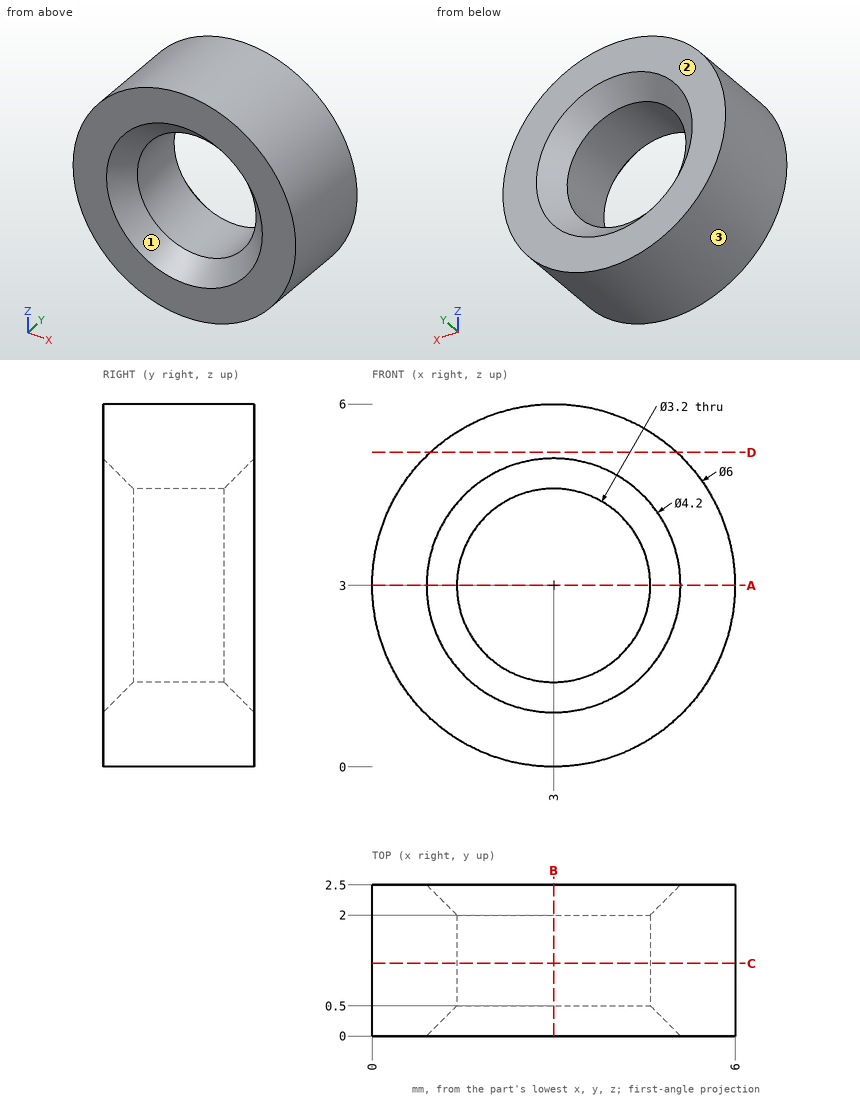
Source: three-view drawing plus pictorial views. Frame: mm from the lowest corner of the part. Give positions to 0.01 mm unless a question says otherwise; leave off trailing zeros. Write each loop counter-clockwise with the first axis right and the second up, starting at its lowest first coordinate (ties: lowest second). Pieces come first, ordered by that corner, then holes.
(1) Ray query, line 1 (Z direction, x = 3, y = 1.3); line 2 (X direction, y = 2.1, z = 2.15); line 3 (Z direction, x = 3.4, y = 2.1). Return the intervals inside material, ascending.
(2) First-contact query: P1, Ø1.5, axis at x = 2, z = 3, coming from the +Y side. Flat tip, straight axial feed; report the tip coordinate or a pass-through.
(3) Cut plane A-A, the plane z = 3. Return loops of the section in (x, y).
(4) Cut plane C-C, the plane y = 1.2. Return loops of the section in (x, z).
(5) Cut plane D-D, the plane z = 5.2. Return loops of the section in (x, y), then the cut area to 3 significant figures.
(6) Cut plane B-B, the plane x = 3. Return loops of the section in (y, z), then the cut area to 3 significant figures.
(7) Mould query, pull axis X, two halves, no side actions, for the marked faces 1, 2 and 3. Classes: released by +X, released by -X, zero draft, split by the parting line, or undercut.
Values follow:
1. line 1: z = 0 to 1.4, 4.6 to 6
1. line 2: x = 0.12 to 1.53, 4.47 to 5.88
1. line 3: z = 0.03 to 1.35, 4.65 to 5.97
2. P1: stops at y = 2.15
3. outline: (0, 0) - (0.9, 0) - (1.4, 0.5) - (1.4, 2) - (0.9, 2.5) - (0, 2.5) - close; (4.6, 0.5) - (5.1, 0) - (6, 0) - (6, 2.5) - (5.1, 2.5) - (4.6, 2) - close
4. outline: circle Ø6 at (3, 3); hole circle Ø3.2 at (3, 3)
5. outline: (0.96, 0) - (5.04, 0) - (5.04, 2.5) - (0.96, 2.5) - close
5. area: 10.2 mm2
6. outline: (0, 0) - (2.5, 0) - (2.5, 0.9) - (2, 1.4) - (0.5, 1.4) - (0, 0.9) - close; (0, 5.1) - (0.5, 4.6) - (2, 4.6) - (2.5, 5.1) - (2.5, 6) - (0, 6) - close
6. area: 6.50 mm2
7. face 1: undercut
7. face 2: zero draft
7. face 3: split by the parting line
